Geometry: final body of the model. Coordinates: model frame, mm. Give positions to 0.01 mm unless a question says otherwise; leave off trailing zeros. Write each loop counter-clockwise with the first axis right and the second up, starting at its lowest first coordinate (ties: lowest second). Pieces come first, ordered by that corner, then holes. Notation, with made-up numbers: M 83.25,14.5 L 134.25,14.5 A6 ccw 134.25,23.5 Z; hole C 80.5,49 d1. An arc over 180 degrees is marked long. Use a Markdown table: item, result. Add a question column.
(1) Material intervals for L1, parallel to Y at x = 25, z = 0.4; L2, parallel to X at y = 24, z = 0.6; L3, parallel to X at y = -1, z = 0.5, sorted ascending.
(2) Cut plane C-C (x = 0). Output: boundary loops of the cut face in (y, z).
(3) Cut plane D-D (x = 55.5). Output: boundary loops of the cut face in (y, z), plus the area to 3 significant figures.
(4) Pin query (flat end, axial travel): pin 1 Ø0.5 at (y, z) = (24, 0.5) entering from +X; pin 2 Ø0.5 at (y, z) = (2.5, 0.5) entering from -X; pin 3 Ø0.5 at (y, z) = (22.5, 0.5) entering from +X; pin 4 Ø4.5 at (x, y) = (75, 25) entering from +Z. Return the tip coordinate at first contact, or that it passes through.
(5) Cut plane B-B (z = 0.3). Output: boundary loops of the cut face in (x, y), plus the area to 3 significant figures.
(6) Cut plane A-A (x = 25). Output: boundary loops of the cut face in (y, z), plus the area to 3 significant figures.
```python
from build123d import *

# Parameters (mm, degrees)
F0_R     = 2
F1_DEPTH = 1
F2_R     = 4.5


with BuildPart() as f1:
    # F0 (on Top) → F1 (new body)
    with BuildSketch(Plane.XY):
        with BuildLine():
            Line((21.818019, 28.181981), (-3.181981, 3.181981))
            ThreePointArc((-3.181981, 3.181981), (-3.181981, -3.181981), (3.181981, -3.181981))
            Line((3.181981, -3.181981), (20.5, 14.136039))
            Line((20.5, 14.136039), (20.5, 0))
            ThreePointArc((20.5, 0), (25, 4.5), (29.5, 0))
            ThreePointArc((29.5, 0), (29.157458, -1.722075), (28.181981, -3.181981))
            Line((28.181981, -3.181981), (45.5, 14.136039))
            Line((45.5, 14.136039), (45.5, 0))
            ThreePointArc((45.5, 0), (50, 4.5), (54.5, 0))
            ThreePointArc((54.5, 0), (54.157458, -1.722075), (53.181981, -3.181981))
            Line((53.181981, -3.181981), (78.181981, 21.818019))
            ThreePointArc((78.181981, 21.818019), (71.818019, 21.818019), (71.818019, 28.181981))
            Line((71.818019, 28.181981), (54.5, 10.863961))
            Line((54.5, 10.863961), (54.5, 25))
            ThreePointArc((54.5, 25), (48.277925, 20.842542), (46.818019, 28.181981))
            Line((46.818019, 28.181981), (29.5, 10.863961))
            Line((29.5, 10.863961), (29.5, 25))
            ThreePointArc((29.5, 25), (23.277925, 20.842542), (21.818019, 28.181981))
        make_face()
        Circle(F0_R, mode=Mode.SUBTRACT)
        with BuildLine():
            ThreePointArc((29.5, 25), (26.722075, 29.157458), (21.818019, 28.181981))
            ThreePointArc((21.818019, 28.181981), (23.277925, 20.842542), (29.5, 25))
        make_face()
        with Locations((25, 25)):
            Circle(F0_R, mode=Mode.SUBTRACT)
        with BuildLine():
            ThreePointArc((29.5, 0), (25, 4.5), (20.5, 0))
            ThreePointArc((20.5, 0), (23.277925, -4.157458), (28.181981, -3.181981))
            ThreePointArc((28.181981, -3.181981), (29.157458, -1.722075), (29.5, 0))
        make_face()
        with Locations((25, 0)):
            Circle(F0_R, mode=Mode.SUBTRACT)
        with BuildLine():
            ThreePointArc((54.5, 0), (50, 4.5), (45.5, 0))
            ThreePointArc((45.5, 0), (48.277925, -4.157458), (53.181981, -3.181981))
            ThreePointArc((53.181981, -3.181981), (54.157458, -1.722075), (54.5, 0))
        make_face()
        with Locations((50, 0)):
            Circle(F0_R, mode=Mode.SUBTRACT)
        with BuildLine():
            ThreePointArc((54.5, 25), (51.722075, 29.157458), (46.818019, 28.181981))
            ThreePointArc((46.818019, 28.181981), (48.277925, 20.842542), (54.5, 25))
        make_face()
        with Locations((50, 25)):
            Circle(F0_R, mode=Mode.SUBTRACT)
        with BuildLine():
            ThreePointArc((79.5, 25), (76.722075, 29.157458), (71.818019, 28.181981))
            ThreePointArc((71.818019, 28.181981), (71.818019, 21.818019), (78.181981, 21.818019))
            ThreePointArc((78.181981, 21.818019), (79.157458, 23.277925), (79.5, 25))
        make_face()
        with Locations((75, 25)):
            Circle(F0_R, mode=Mode.SUBTRACT)
    extrude(amount=F1_DEPTH)

    # F2
    f2_edges = [f1.edges().sort_by_distance(p)[0] for p in [
        (20.5, 14.136039, 0.5),
        (45.5, 14.136039, 0.5),
        (29.5, 10.863961, 0.5),
        (54.5, 10.863961, 0.5),
    ]]
    fillet(f2_edges, radius=F2_R)


solid = f1.part
```
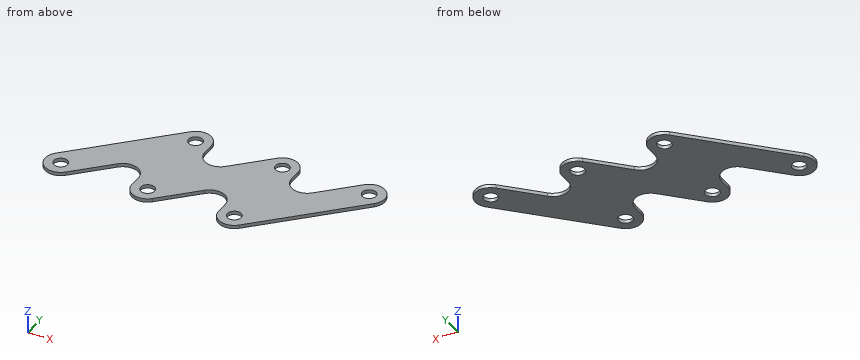
Answer list:
| question | item | result |
|---|---|---|
| 1 | L1 | -4.5 to -2, 2 to 23, 27 to 29.5 |
| 1 | L2 | 17.64 to 23.27, 26.73 to 29.5, 42.64 to 48.27, 51.73 to 54.5, 67.64 to 73.27, 76.73 to 79.39 |
| 1 | L3 | -4.39 to -1.73, 1.73 to 5.36, 20.61 to 23.27, 26.73 to 30.36, 45.61 to 48.27, 51.73 to 55.36 |
| 2 | outline | M -4.5,0 L -2,0 L -2,1 L -4.5,1 Z; M 2,0 L 6.36,0 L 6.36,1 L 2,1 Z |
| 3 | outline | M -0.86,0 L 18.9,0 L 18.9,1 L -0.86,1 Z |
| 3 | area | 19.8 mm² |
| 4 | pin 1 | x = 79.44 |
| 4 | pin 2 | x = -3.9 |
| 4 | pin 3 | x = 78.9 |
| 4 | pin 4 | z = 1 |
| 5 | outline | M -3.18,3.18 A4.5 ccw 3.18,-3.18 L 12.82,6.45 A4.5 cw 20.5,3.27 L 20.5,0 A4.5 ccw 28.18,-3.18 L 37.82,6.45 A4.5 cw 45.5,3.27 L 45.5,0 A4.5 ccw 53.18,-3.18 L 78.18,21.82 A4.5 ccw 79.5,25 A4.5 ccw 71.82,28.18 L 62.18,18.55 A4.5 cw 54.5,21.73 L 54.5,25 A4.5 ccw 46.82,28.18 L 37.18,18.55 A4.5 cw 29.5,21.73 L 29.5,25 A4.5 ccw 21.82,28.18 Z; hole C 0,0 d4; hole C 25,0 d4; hole C 25,25 d4; hole C 50,0 d4; hole C 50,25 d4; hole C 75,25 d4 |
| 5 | area | 1,390 mm² |
| 6 | outline | M -4.5,0 L -2,0 L -2,1 L -4.5,1 Z; M 2,0 L 23,0 L 23,1 L 2,1 Z; M 27,0 L 29.5,0 L 29.5,1 L 27,1 Z |
| 6 | area | 26.0 mm² |
